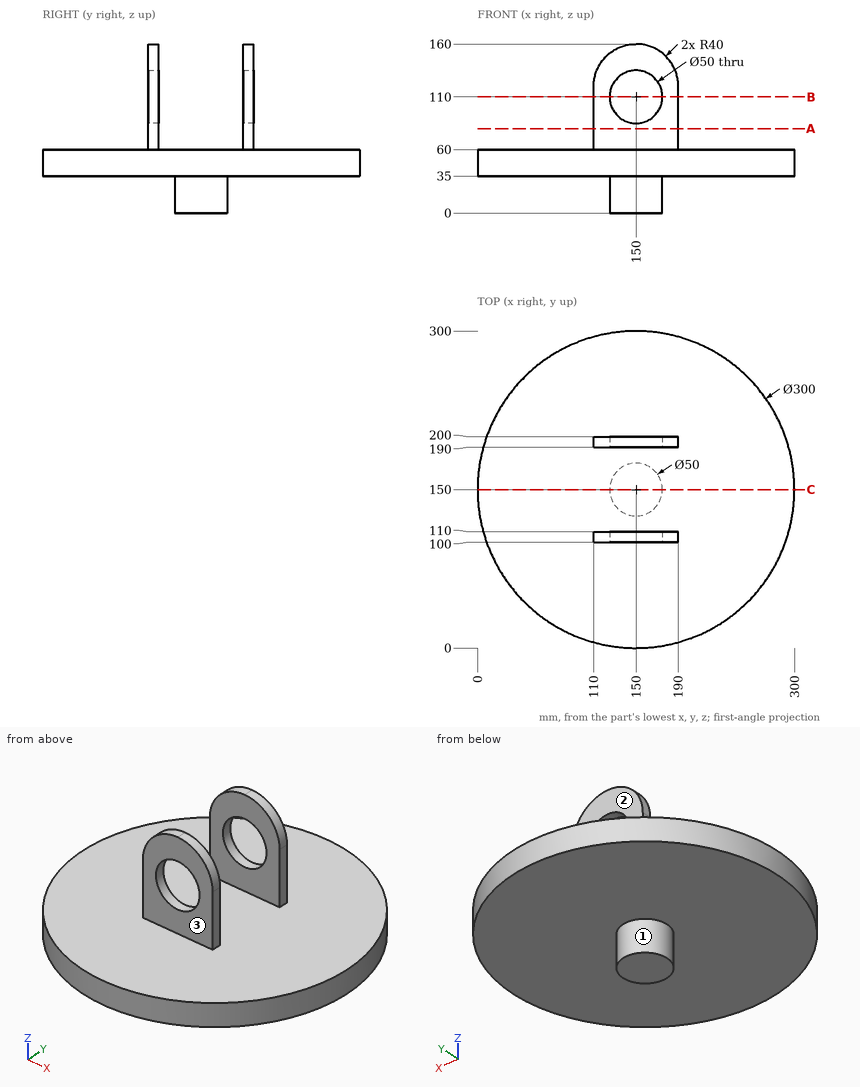
Here's the drawing with two shaded views (mm, measured from the low corner). I have some questions. A direction names the side the tool comes from. Give positions to 0.01 mm unless a question says otherwise; leave off trailing zeros. Loops run counter-clockwise (first coordinate to the right, second up) from the corner with the lowest first, then second, coordinate; pieces in that order, holes last. Notation, with made-up numbers: M 77,53.25 L 110,53.25 A19 ccw 110,82.25 Z; hole C 11,-23.5 d6. An arc over 180 degrees is marked long. One line per item, written item: value. Start each with the question number.
1) If I drill on line 1 (X direction, y = 104.75, z = 110); line 2 (Z direction, x = 150, y = 194); line 3 (Z direction, x = 214, y = 164.5), over which ranges is the centre line in solid material (lowest first)? Write a range as [from, to].
2) If we section it at A-A, the plane z = 80: Write out the boundary of the cut face in (x, y), and give its area (3 significant figures).
3) If we section it at C-C, the plane y = 150: Write out the boundary of the cut face in (x, z), and give its area (3 significant figures).
4) I'm going to push flat-ended pins straight in: pin 1 (2 mm diameter, centred on x = 32, z = 53, fed in from +Y); pin 2 (8 mm diameter, centred on x = 127, z = 86, fed in from +Y); pin 3 (5 mm diameter, centred on y = 106, z = 96.5, fed in from +X); pin 4 (24 mm diameter, centred on x = 154.5, z = 109.5, fed in from -Y). Where does each tip first touch, or does it pass through?
5) On a 3-axis mill with a long thin cutter (end or side, diameter ignored), from which of +Z, -Z, +X, -X, +Y, -Y can I reach the whole of each face in a straight line? I mean the marked faces 1, 2 and 3. Say none if no direction works.
6) If we section it at B-B, the plane z = 110: Write out the boundary of the cut face in (x, y), and give its area (3 significant figures).
Completed:
1. line 1: x = [110, 125], [175, 190]
1. line 2: z = [35, 85], [135, 160]
1. line 3: z = [35, 60]
2. outline: M 110,100 L 190,100 L 190,110 L 110,110 Z; M 110,190 L 190,190 L 190,200 L 110,200 Z
2. area: 1,600 mm^2
3. outline: M 0,35 L 125,35 L 125,0 L 175,0 L 175,35 L 300,35 L 300,60 L 0,60 Z
3. area: 9,250 mm^2
4. pin 1: stops at y = 243.87
4. pin 2: stops at y = 200
4. pin 3: stops at x = 190
4. pin 4: passes through
5. face 1: -Z
5. face 2: +Z, +X, -X, +Y
5. face 3: +Z, +X, -X, -Y
6. outline: M 110,100 L 125,100 L 125,110 L 110,110 Z; M 110,190 L 125,190 L 125,200 L 110,200 Z; M 175,100 L 190,100 L 190,110 L 175,110 Z; M 175,190 L 190,190 L 190,200 L 175,200 Z
6. area: 600 mm^2
